The model under review builds one solid part; all positions refer to its coordinate system, in mm. A direction names the side the tool comes from. Give positions to 0.01 mm unless a question says otherwise; leave off trailing zeros. Write each loop counter-clockwise with the first axis right and the second up, starting at its lowest first coordinate (ties: lowest second). Pieces come first, ordered by that corner, then holes.
from build123d import *

# Parameters (mm, degrees)
F1_DEPTH = 76.2
F2_R     = 19.05
F3_DEPTH = 76.2


with BuildPart() as f1:
    # F0 (on Front) → F1 (new body)
    with BuildSketch(Plane.XZ):
        Polygon((25.4, 0), (0, 0), (0, 50.8), (-25.4, 50.8), (-25.4, -25.4), (25.4, -25.4), align=None)
    extrude(amount=F1_DEPTH)

    # F2 (on face) → F3 (join)
    with BuildSketch(Plane.YZ):
        with Locations((-38.1, 25.4)):
            Circle(F2_R)
    extrude(amount=F3_DEPTH)


solid = f1.part
1) Consider section A-A, the plane x = 5. Give the boundary of the cut face in (y, z).
2) Consider section C-C, the plane y = -38.1. Give the boundary of the cut face in (x, z).
3) To check wall thickness, follow probe 1 along Z at (x, y) = (21.5, -38); probe 2 along X at (y, z) = (-72, 24). State the ranges of each line that lie inside material, in increasing order.
4) Consider section B-B, the plane z = 25.4. Give the boundary of the cut face in (x, y), then the cut area to 3 significant figures.
5) Tool access review of faces 5 (the flat face through (-6, -76.2, 5)), 6 (the flat face through (25.4, -38, -13)), 7 (the flat face through (13, -38, 0)): name each direction out of +Z, -Z, +X, -X, +Y, -Y from which nothing blocks a thin tool from reaching the whole face with its end or side.
6) Consider section D-D, the plane x = 27. Give the boundary of the cut face in (y, z), then the cut area to 3 significant figures.
7) The part is to be moulded in two halves that separate along Z. For faces 1 (the flat face through (0, -29, 8)), 2 (the flat face through (76.2, -38, 26)), 3 (the flat face through (0, -38, -25.4)), 4 (the cylindrical face through (37.567, -42.23, 6.803)), say which applies: +Z half, -Z half, draft (parallel to the pull), parting line (faces both ways), or undercut.
8) Insertion check: pin 1 (2 mm diameter, centred on y = -31, z = -5, fed in from +X); pin 2 (1.5 mm diameter, centred on x = 61, z = 37, fed in from +Y); pin 3 (1.5 mm diameter, centred on x = 16, z = 14, fed in from +Y). Each pin has a flat end and moves straight along its axis. Give the tip position at first contact, or say it passes through.
Answer block:
1. outline: (-76.2, -25.4) - (0, -25.4) - (0, 0) - (-76.2, 0) - close; circle Ø38.1 at (-38.1, 25.4)
2. outline: (-25.4, -25.4) - (25.4, -25.4) - (25.4, 0) - (0, 0) - (0, 6.35) - (76.2, 6.35) - (76.2, 44.45) - (0, 44.45) - (0, 50.8) - (-25.4, 50.8) - close
3. probe 1: z = -25.4 to 0, 6.35 to 44.45
3. probe 2: x = -25.4 to 0
4. outline: (-25.4, -76.2) - (0, -76.2) - (0, -57.15) - (76.2, -57.15) - (76.2, -19.05) - (0, -19.05) - (0, 0) - (-25.4, 0) - close
4. area: 4,840 mm2
5. face 5: +Z, -Z, +X, -X, -Y
5. face 6: -Z, +X, +Y, -Y
5. face 7: +X, +Y, -Y
6. outline: circle Ø38.1 at (-38.1, 25.4)
6. area: 1,140 mm2
7. face 1: undercut
7. face 2: draft
7. face 3: -Z half
7. face 4: undercut
8. pin 1: stops at x = 25.4
8. pin 2: stops at y = -22.44
8. pin 3: stops at y = -22.31
